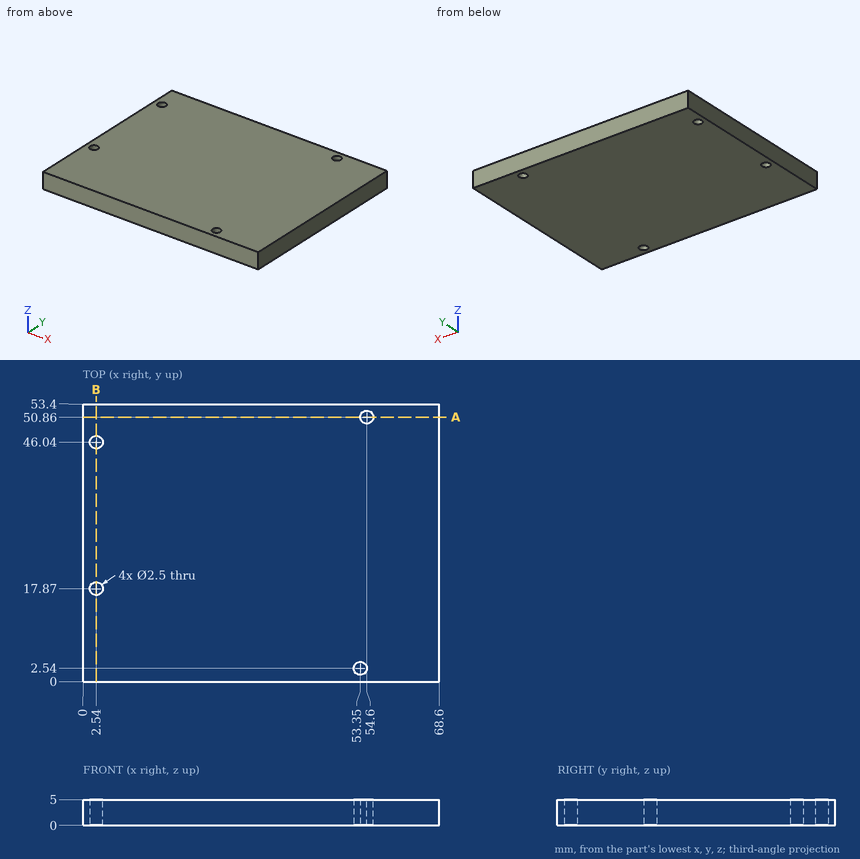
Geometry check sheet. Reference: drawing and pictorial views, mm from the part's lowest x, y, z. Coordinates: 2 decimals unless noted, no trailing zeros. Order: outer loops, then holes, each group sorted by start corner. A loop starts at its lowest first (then second) coordinate and runs counter-clockwise, first axis right, second up. Notation, with made-up numbers: (5.25, -7.5) -> (21.25, -7.5) arc R20 cw to (21.25, 6.5) -> close; hole circle Ø10 at (36, -5.5). An arc over 180 degrees is marked (long way). Use CSV: the item, a comma, the result in double quotes. Start each with the question number.
Q1. Section check A-A, the plane y = 50.86. Record the cut outline in (x, z).
Q2. Thickness scan on line 1 along Y through (x, z) = (2.54, 3.6); line 2 along X through (y, z) = (46.04, 3.6); line 3 along X through (y, z) = (50.86, 1.55). Record the ranges inside material, lowest first.
Q3. Section check B-B, the plane x = 2.54. Record the cut outline in (y, z).
Returned:
1,outline,"(0, 0) -> (53.35, 0) -> (53.35, 5) -> (0, 5) -> close; (55.85, 0) -> (68.6, 0) -> (68.6, 5) -> (55.85, 5) -> close"
2,line 1,"y = 0 to 16.62, 19.12 to 44.79, 47.29 to 53.4"
2,line 2,"x = 0 to 1.29, 3.79 to 68.6"
2,line 3,"x = 0 to 53.35, 55.85 to 68.6"
3,outline,"(0, 0) -> (16.62, 0) -> (16.62, 5) -> (0, 5) -> close; (19.12, 0) -> (44.79, 0) -> (44.79, 5) -> (19.12, 5) -> close; (47.29, 0) -> (53.4, 0) -> (53.4, 5) -> (47.29, 5) -> close"
